Autodesk Fusion 360 part; units mm, degrees
sketch "Sketch1" plane through (0, 0, 0) normal (0, 0, 1) x (1, 0, 0)
  line L0 (0, 0) -> (406.4, 0)
  line L1 (406.4, 0) -> (406.4, 711.2)
  line L2 (406.4, 711.2) -> (0, 711.2)
  line L3 (0, 711.2) -> (0, 0)
  arc A0 (0, 635) -> (76.2, 711.2) centre (0, 711.2) ccw
  arc A1 (330.2, 711.2) -> (406.4, 635) centre (406.4, 711.2) ccw
  arc A2 (76.2, 0) -> (0, 76.2) centre (0, 0) ccw
  arc A3 (406.4, 76.2) -> (330.2, 0) centre (406.4, 0) ccw
  dimension "d1" = 406.4
  dimension "d2" = 711.2
  dimension "d5" = 152.4
  dimension "d6" = 152.4
  dimension "d7" = 152.4
  dimension "d8" = 152.4
extrude "Extrude1" add sketch "Sketch1" along normal blind 5.715 contours L0 L1 L2 L3 A0 A1 A2 A3 makes body 1
copy_body "Body->Comp1" bodies 1 removing the originals makes body 2 in component "Component"
component "Component" placed x (1, 0, 0) y (0, 1, 0) z (0, 0, 1) at (0, 0, 0)
Read the model definition and answer for the solid it produces. Units are mm, in the model's axes. Coordinates: 2 decimals unless noted, no trailing zeros. Order: outer loops, then holes, each group sorted by start corner. A loop starts at its lowest first (then second) coordinate and runs counter-clockwise, first axis right, second up. Notation, with made-up numbers: (23, -15) - (27, -15) arc R32 ccw to (27, 11) - close; hole circle Ø8 at (87.25, 51.25). An arc over 180 degrees is marked (long way). Answer as a JSON object with one key per item and string values. Group by question number.
Item 1: Consider probe 1 along Y at (x, z) = (42.5, 3.75); probe 2 along X at (y, z) = (68, 5.5). Determine where each line is inside the solid, lowest interval first. Write a range as from..to.
Item 2: The mould has two halves that part along X. Classify faces 1 (the face through (351.929, 53.286, 2.817)), 2 (the face through (200, 361, 5.715)), 3 (the face through (53.286, 54.471, 2.817)): +X half, -X half, draft (parallel to the pull), parting line (faces both ways), or undercut.
Item 3: Section A-A (z = 2.45) is taken. Give the vertices of the cut face in (x, y), plus the area to 3 significant figures.
Item 4: A flat-ended cylindrical pin translates along its axis: P1, Ø3, axis at x = 344.5, z = 5, coming from the -Y side. Find the tip coordinate at first contact, or state that the pin passes through.
Item 5: Section B-B (y = 46.5) is taken. Give the vertices of the cut face in (x, z) (3 decimals).
Item 6: Section C-C (x = 56.5) is taken. Give the vertices of the cut face in (y, z) (3 decimals).
Results are:
{
 "1": {"probe 1": "y = 63.25..647.95", "probe 2": "x = 34.39..372.01"},
 "2": {"face 1": "+X half", "face 2": "draft", "face 3": "-X half"},
 "3": {"outline": "(0, 76.2) arc R76.2 cw to (76.2, 0) - (330.2, 0) arc R76.2 cw to (406.4, 76.2) - (406.4, 635) arc R76.2 cw to (330.2, 711.2) - (76.2, 711.2) arc R76.2 cw to (0, 635) - close", "area": "271,000 mm^2"},
 "4": {"P1": "stops at y = 42.27"},
 "5": {"outline": "(60.367, 0) - (346.033, 0) - (346.033, 5.715) - (60.367, 5.715) - close"},
 "6": {"outline": "(51.129, 0) - (660.071, 0) - (660.071, 5.715) - (51.129, 5.715) - close"}
}
